Could you check a few things on this model? Use its own coordinates, in mm. Face numbers are marked on the shaded views. Give positions to 0.01 mm unless a question says otherwise; leave off trailing zeros. Loops run counter-clockwise (first coordinate to the right, second up) from the corner with the lowest first, then second, coordinate; pieces in that order, holes last. Notation, with made-up numbers: (17, 18.5) - (43, 18.5) arc R27 cw to (43, 53.5) - close; hole circle Ø5 at (-11.5, 61.5). An arc over 180 degrees is marked (long way). One line per item, written item: value. Start each with the question number.
Q1. If I drill on line 1 (Y direction, x = 0, z = 3.75) (3 decimals); line 2 (Y direction, x = -5, z = 3); line 3 (Y direction, x = 22, z = 1.25), over which ranges is the centre line in solid material (lowest first)? Write a range as from..to.
Q2. I want a section at A-A (x = 0). Please give me the cut outline in (y, z) (3 decimals), then the cut area to 3 significant figures.
Q3. I want a section at B-B (z = 4). Count the separate pieces of the cut face and the enclosed holes in it, then the cut area to 3 significant figures.
Q4. I'm going to push flat-ended pins straight in: P1, Ø1.5, axis at y = 29, z = 5, coming from the -X side; P2, Ø12, axis at x = -30.5, y = -19.5, coming from the +Z side; P3, Ø2.5, axis at y = 23, z = 3, coming from the +X side (3 decimals); P4, Ø4, axis at y = 9.5, z = 6, coming from the -X side. Where does each tip first touch, or does it pass through?
Q5. If we mould it in two halves opening along Y, with no side actions, what happens to the marked faces 1 and 2? For each: released by +Y, released by -Y, zero draft, split by the parting line, or undercut.
```python
from build123d import *

# Parameters (mm, degrees)
F0_R     = 11.025
F1_DEPTH = 7
F2_R     = 2


with BuildPart() as f1:
    # F0 (on Top) → F1 (new body)
    with BuildSketch(Plane.XY):
        with BuildLine():
            ThreePointArc((14.025, 27.75), (0, 41.775), (-14.025, 27.75))
            Line((-14.025, 27.75), (-14.025, 10.984089))
            ThreePointArc((-14.025, 10.984089), (-14.694873, 8.484089), (-16.525, 6.653962))
            Line((-16.525, 6.653962), (-31.044705, -1.728994))
            ThreePointArc((-31.044705, -1.728994), (-36.178211, -20.8875), (-17.019705, -26.021006))
            Line((-17.019705, -26.021006), (-2.5, -17.638051))
            ThreePointArc((-2.5, -17.638051), (0, -16.968178), (2.5, -17.638051))
            Line((2.5, -17.638051), (17.019705, -26.021006))
            ThreePointArc((17.019705, -26.021006), (36.178211, -20.8875), (31.044705, -1.728994))
            Line((31.044705, -1.728994), (16.525, 6.653962))
            ThreePointArc((16.525, 6.653962), (14.694873, 8.484089), (14.025, 10.984089))
            Line((14.025, 10.984089), (14.025, 27.75))
        make_face()
        with Locations((-24.032205, -13.875)):
            Circle(F0_R, mode=Mode.SUBTRACT)
        with BuildLine():
            Line((-1.158934, -13.977035), (-11.348271, -19.859851))
            ThreePointArc((-11.348271, -19.859851), (-10.014308, -14.321322), (-10.993239, -8.709152))
            ThreePointArc((-10.993239, -8.709152), (-6.622422, -12.363015), (-1.158934, -13.977035))
        make_face(mode=Mode.SUBTRACT)
        with BuildLine():
            ThreePointArc((-12.683934, 5.984851), (-14.017896, 0.446322), (-13.038966, -5.165848))
            ThreePointArc((-13.038966, -5.165848), (-17.409783, -1.511985), (-22.873271, 0.102035))
            Line((-22.873271, 0.102035), (-12.683934, 5.984851))
        make_face(mode=Mode.SUBTRACT)
        with BuildLine():
            ThreePointArc((1.158934, -13.977035), (6.622422, -12.363015), (10.993239, -8.709152))
            ThreePointArc((10.993239, -8.709152), (10.014308, -14.321322), (11.348271, -19.859851))
            Line((11.348271, -19.859851), (1.158934, -13.977035))
        make_face(mode=Mode.SUBTRACT)
        with Locations((24.032205, -13.875)):
            Circle(F0_R, mode=Mode.SUBTRACT)
        Circle(F0_R, mode=Mode.SUBTRACT)
        with BuildLine():
            Line((12.683934, 5.984851), (22.873271, 0.102035))
            ThreePointArc((22.873271, 0.102035), (17.409783, -1.511985), (13.038966, -5.165848))
            ThreePointArc((13.038966, -5.165848), (14.017896, 0.446322), (12.683934, 5.984851))
        make_face(mode=Mode.SUBTRACT)
        with BuildLine():
            ThreePointArc((-11.525, 19.757816), (-7.395474, 15.833307), (-2.045727, 13.875))
            ThreePointArc((-2.045727, 13.875), (-4.610881, 13.245392), (-7.0125, 12.146006))
            Line((-7.0125, 12.146006), (-11.525, 9.540713))
            Line((-11.525, 9.540713), (-11.525, 19.757816))
        make_face(mode=Mode.SUBTRACT)
        with BuildLine():
            ThreePointArc((7.0125, 12.146006), (4.610881, 13.245392), (2.045727, 13.875))
            ThreePointArc((2.045727, 13.875), (7.395474, 15.833307), (11.525, 19.757816))
            Line((11.525, 19.757816), (11.525, 9.540713))
            Line((11.525, 9.540713), (7.0125, 12.146006))
        make_face(mode=Mode.SUBTRACT)
        with Locations((0, 27.75)):
            Circle(F0_R, mode=Mode.SUBTRACT)
    extrude(amount=F1_DEPTH)

    # F2
    f2_edges = [f1.edges().sort_by_distance(p)[0] for p in [
        (-36.178211, -20.8875, 7),
        (-9.759852, -21.829529, 7),
        (0, -16.968178, 7),
        (9.759852, -21.829529, 7),
        (36.178211, -20.8875, 7),
        (23.784852, 2.462484, 7),
        (14.694873, 8.484089, 7),
        (-23.784852, 2.462484, 7),
        (-14.694873, 8.484089, 7),
        (0, 41.775, 7),
        (14.025, 19.367044, 7),
        (-23.784852, 2.462484, 0),
        (-36.178211, -20.8875, 0),
    ]]
    fillet(f2_edges, radius=F2_R)


solid = f1.part
```
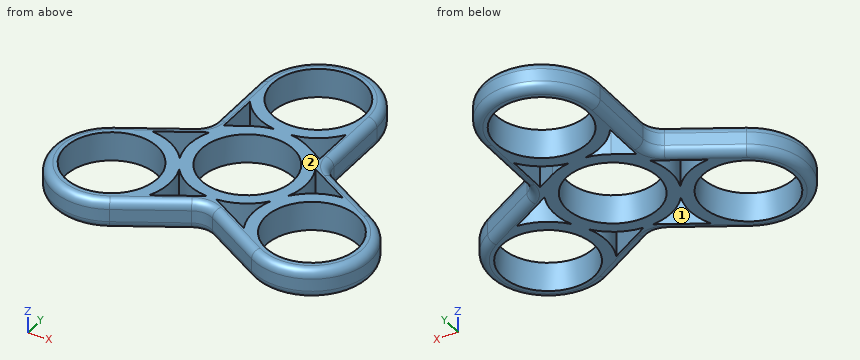
Worked answers:
1. line 1: y = -16.968..-11.025, 11.025..16.725, 38.775..41.775
1. line 2: y = -19.08..-16.19, -13.1..-9.83, 9.83..13.1, 14.65..17.92, 37.58..40.85
1. line 3: y = -27.6..-24.71, -3.04..0, 0.61..3.32
2. outline: (-16.968, 2) arc R2 ccw to (-14.968, 0) - (-11.025, 0) - (-11.025, 7) - (-14.968, 7) arc R2 ccw to (-16.968, 5) - close; (11.025, 0) - (16.725, 0) - (16.725, 7) - (11.025, 7) - close; (38.775, 0) - (39.775, 0) arc R2 ccw to (41.775, 2) - (41.775, 5) arc R2 ccw to (39.775, 7) - (38.775, 7) - close
2. area: 99.1 mm²
3. separate pieces: 1
3. enclosed holes: 10
3. area: 1,170 mm²
4. P1: stops at x = -14.02
4. P2: stops at z = 7
4. P3: stops at x = 14.025
4. P4: stops at x = -15.3
5. face 1: undercut
5. face 2: zero draft
